```python
from build123d import *

# Parameters (mm, degrees)
SKETCH_1_R        = 8.975
SKETCH_1_R_2      = 6.8
EXTRUDE_1_DEPTH   = 11.75
EXTRUDE_1_2_DEPTH = 11.75
SKETCH_3_R        = 8.975
EXTRUDE_4_DEPTH   = 3.7


with BuildPart() as part:
    # Sketch 1 → Extrude 1 (new, symmetric)
    with BuildSketch(Plane(origin=(0, 0, 0), x_dir=(0, 0, -1), z_dir=(1, 0, 0))):
        with Locations((-19.05, 0)):
            Circle(SKETCH_1_R)
        with Locations((-19.05, 0)):
            Circle(SKETCH_1_R_2, mode=Mode.SUBTRACT)
    extrude(amount=EXTRUDE_1_DEPTH, both=True)



with BuildPart() as body_2:
    # Sketch 1 → Extrude 1 2 (new, symmetric)
    with BuildSketch(Plane(origin=(0, 0, 0), x_dir=(0, 0, -1), z_dir=(1, 0, 0))):
        with Locations((19.05, 0)):
            Circle(SKETCH_1_R)
        with Locations((19.05, 0)):
            Circle(SKETCH_1_R_2, mode=Mode.SUBTRACT)
    extrude(amount=EXTRUDE_1_2_DEPTH, both=True)


with BuildPart() as part_1:
    add(part.part)

    add(body_2.part)  # Extrude 4 merges body 2
    # Sketch 3 → Extrude 4 (add)
    with BuildSketch(Plane(origin=(11.75, 0, 0), x_dir=(0, 0, -1), z_dir=(1, 0, 0))):
        with BuildLine():
            ThreePointArc((12.929864253, -12.813428052), (33.25, 0), (12.929864253, 12.813428052))
            ThreePointArc((12.929864253, 12.813428052), (0, 9.884050697), (-12.929864253, 12.813428052))
            ThreePointArc((-12.929864253, 12.813428052), (-33.25, 0), (-12.929864253, -12.813428052))
            ThreePointArc((-12.929864253, -12.813428052), (0, -9.884050697), (12.929864253, -12.813428052))
        make_face()
        with Locations((-19.05, 0)):
            Circle(SKETCH_3_R, mode=Mode.SUBTRACT)
        with Locations((19.05, 0)):
            Circle(SKETCH_3_R, mode=Mode.SUBTRACT)
    extrude_4 = extrude(amount=-EXTRUDE_4_DEPTH)

    # Mirror 10: Extrude 4 across plane
    add(extrude_4.mirror(Plane(origin=(0, 0, 0), x_dir=(0, 0, 1), z_dir=(1, 0, 0))))


solid = part_1.part
```
Input: part model. Units: mm. Frame: model coordinates. A direction names the side the tool comes from. Give positions to 0.01 mm unless a question says otherwise; leave off trailing zeros. Order: outer loops, then holes, each group sorted by start corner. A loop starts at its lowest first (then second) coordinate and runs counter-clockwise, first axis right, second up.
1. Draft query along X for faces 3 (the face through (-11.75, 0, 0)), 4 (the face through (9.926, -0.401, -33.244)), 5 (the face through (0.113, 0.395, 28.016)). Return one class per face: released by +X, released by -X, zero draft, split by the parting line, or undercut.
Computed:
face 3: released by -X
face 4: zero draft
face 5: undercut
2. Set-up query: faces 1 (the face through (9.926, 9.885, -0.187)), 2 (the face through (8.05, 0, 0)). Return all of +Z, -Z, +X, -X, +Y, -Y with unobstructed straight access to the full face (end or side cutting, diameter ignored); none if empty.
Computed:
face 1: +X, -X, +Y
face 2: none
3. Pin query (flat end, axial travel): pin 1 Ø10 at (x, y) = (-7, -10.5) entering from +Z; pin 2 Ø10 at (x, y) = (9, 3) entering from +Z; pin 3 Ø8 at (x, y) = (-1, 4.5) entering from +Z; pin 4 Ø12 at (x, z) = (-6, -2.5) entering from -Y. Return the tip coordinate at first contact, or that it passes through.
Computed:
pin 1: stops at z = 32.09
pin 2: stops at z = 33.25
pin 3: stops at z = 28.01
pin 4: stops at y = -11.01
4. Line query: probe 1 along X at (y, z) = (7.75, -6); probe 2 along Z at (x, y) = (-5.5, -4); probe 3 along Y at (x, z) = (3.75, -19.05) (3 decimals). Output: solid intervals per line, ascending.
Computed:
probe 1: x = -11.75 to -8.05, 8.05 to 11.75
probe 2: z = -27.08 to -24.55, -13.55 to -11.02, 11.02 to 13.55, 24.55 to 27.08
probe 3: y = -8.975 to -6.8, 6.8 to 8.975
5. Cut plane D-D (y = 12). Return loops of the section in (x, z).
Computed:
outline: (-11.75, -26.64) - (-8.05, -26.64) - (-8.05, -11.07) - (-11.75, -11.07) - close; (-11.75, 11.07) - (-8.05, 11.07) - (-8.05, 26.64) - (-11.75, 26.64) - close; (8.05, -26.64) - (11.75, -26.64) - (11.75, -11.07) - (8.05, -11.07) - close; (8.05, 11.07) - (11.75, 11.07) - (11.75, 26.64) - (8.05, 26.64) - close
6. Cut plane A-A (y = 0). Return loops of the section in (x, z) (3 decimals), and give its area (3 significant figures).
Computed:
outline: (-11.75, -33.25) - (-8.05, -33.25) - (-8.05, -28.025) - (8.05, -28.025) - (8.05, -33.25) - (11.75, -33.25) - (11.75, -25.85) - (-11.75, -25.85) - close; (-11.75, -12.25) - (11.75, -12.25) - (11.75, 12.25) - (-11.75, 12.25) - close; (-11.75, 25.85) - (11.75, 25.85) - (11.75, 33.25) - (8.05, 33.25) - (8.05, 28.025) - (-8.05, 28.025) - (-8.05, 33.25) - (-11.75, 33.25) - close; hole (-8.05, -10.075) - (8.05, -10.075) - (8.05, 10.075) - (-8.05, 10.075) - close
area: 431 mm2
7. Cut plane C-C (x = 1). Return loops of the section in (y, z) (3 decimals), and give its area (3 significant figures).
Computed:
outline: circle Ø17.95 at (0, -19.05); circle Ø17.95 at (0, 19.05); hole circle Ø13.6 at (0, -19.05); hole circle Ø13.6 at (0, 19.05)
area: 216 mm2
8. Cut plane B-B (z = -19.05). Return loops of the section in (x, y) (3 decimals).
Computed:
outline: (-11.75, -14.2) - (-8.05, -14.2) - (-8.05, -8.975) - (8.05, -8.975) - (8.05, -14.2) - (11.75, -14.2) - (11.75, -6.8) - (-11.75, -6.8) - close; (-11.75, 6.8) - (11.75, 6.8) - (11.75, 14.2) - (8.05, 14.2) - (8.05, 8.975) - (-8.05, 8.975) - (-8.05, 14.2) - (-11.75, 14.2) - close
